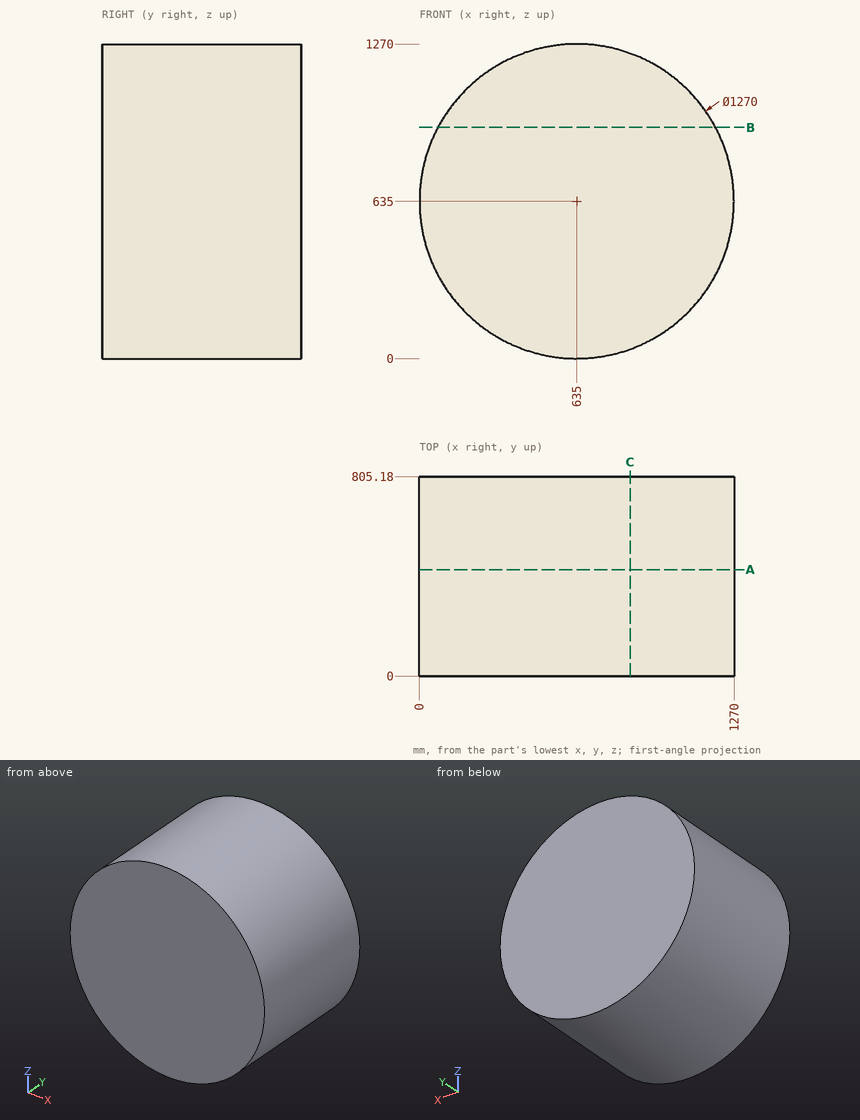
Check sheet for the drawn part. Datum: minimum x, y, z corner. Units: mm. Give positions to 0.01 mm unless a question says otherwise; leave off trailing zeros. Loops run counter-clockwise (first coordinate to the right, second up) from the corner with the lowest first, then second, coordinate; pieces in that order, holes last. Notation, with made-up numbers: M -32.75,42 L 10.25,42 A21 ccw 10.25,80 Z; hole C 23.5,33 d3. An arc over 180 degrees is marked long. Return JSON: item names as keys, results as strings.
1) Section check B-B, the plane z = 933. Enter the section's corners in (x, y), and give its area (3 significant figures).
Findings:
{"outline": "M 74.27,0 L 1195.73,0 L 1195.73,805.18 L 74.27,805.18 Z", "area": "903,000 mm2"}
2) Gauge pin test, flat ends, axial feed: P1, Ø2, axis at y = 357.5, z = 890.5, coming from the +X side; P2, Ø1.5, axis at x = 1072, y = 349.5, coming from the -Z side; P3, Ø12, axis at y = 346, z = 1131.5, coming from the +X side. Record the tip position at first contact, or that the pin passes through.
Findings:
{"P1": "stops at x = 1216.77", "P2": "stops at z = 173.58", "P3": "stops at x = 1038.28"}
3) Material ranges on L1, parallel to Z at x = 757, y = 632.5; L2, parallel to X at y = 412, z = 98.5; L3, parallel to Z at x = 748, y = 405, recorded low to high. Write a range as [from, to].
Findings:
{"L1": "z = [11.83, 1258.17]", "L2": "x = [295.3, 974.7]", "L3": "z = [10.14, 1259.86]"}
4) Section check A-A, the plane y = 429. Enter the section's corners in (x, z).
Findings:
{"outline": "C 635,635 d1270"}
5) Section check C-C, the plane x = 851. Enter the section's corners in (y, z).
Findings:
{"outline": "M 0,37.87 L 805.18,37.87 L 805.18,1232.13 L 0,1232.13 Z"}
